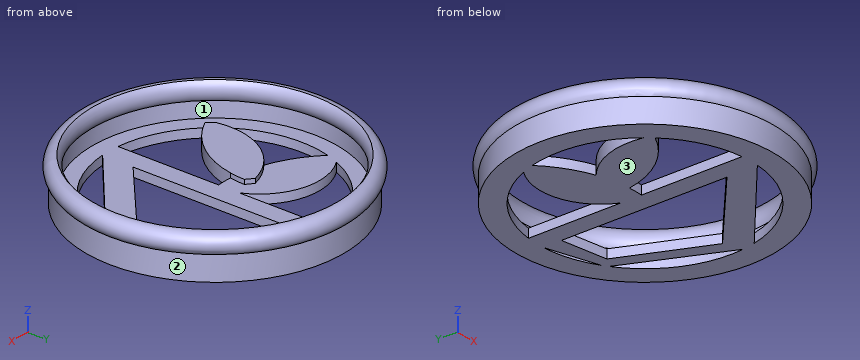
from build123d import *

# Parameters (mm, degrees)
F3_DEPTH = 2
F4_DEPTH = 1


# Not quite as in the source:
# - a feature names something its author has since deleted; it is built from what else it names


with BuildPart() as f1:
    # F0 (on Front) → F1 (revolve)
    with BuildSketch(Plane.XZ):
        Polygon((-29, 0), (-24, 0), (-24, 2), (-27.5, 2), (-27.5, 5.5), (-29, 5.5), align=None)
        with BuildLine():
            ThreePointArc((-27.5, 9.6169896424), (-29.7772258205, 8.1149302096), (-29, 5.5))
            Line((-29, 5.5), (-27.5, 5.5))
            ThreePointArc((-27.5, 5.5), (-26.6610115833, 7.5584948212), (-27.5, 9.6169896424))
        make_face()
    revolve(axis=Axis((0, 0, 2.7132770047), (0, 0, -1)))

    # F2 (on face) → F3 (join)
    with BuildSketch(Plane.XY.offset(2)):
        with BuildLine():
            Line((23.5357220544, -2.0133285341), (14.1158952872, 19.40982999))
            ThreePointArc((14.1158952872, 19.40982999), (13.5624984717, 19.8004705804), (12.9982976167, 20.1753378923))
            Line((12.9982976167, 20.1753378923), (1.5001369464, 23.9530705577))
            ThreePointArc((1.5001369464, 23.9530705577), (-0.61185618, 23.9921993993), (-2.7191094967, 23.8454700844))
            Line((-2.7191094967, 23.8454700844), (-2.7191094967, 3.205855377))
            Line((-2.7191094967, 3.205855377), (-2.7191094967, -1.398249995))
            Line((-2.7191094967, -1.398249995), (-2.7191094967, -23.8454700844))
            ThreePointArc((-2.7191094967, -23.8454700844), (-0.6587764532, -23.9909569127), (1.406435812, -23.9587549407))
            Line((1.406435812, -23.9587549407), (23.3430031088, -5.5771144744))
            ThreePointArc((23.3430031088, -5.5771144744), (23.6412294167, -4.1342800662), (23.8503615327, -2.6758652355))
            Line((23.8503615327, -2.6758652355), (23.5357220544, -2.0133285341))
        make_face()
        Polygon((1.5001369464, -17.0947052702), (1.5001369464, 19.8581963794), (11.7461745714, 17.9819713885), (19.9739150703, -1.2165056542), align=None, mode=Mode.SUBTRACT)
        with BuildLine():
            ThreePointArc((-2.7191094967, 3.205855377), (-11.036038033, 10.667911986), (-22.125575094, 9.2983292455))
            ThreePointArc((-22.125575094, 9.2983292455), (-22.6453594845, 7.9490687392), (-23.0829490937, 6.5709558771))
            ThreePointArc((-23.0829490937, 6.5709558771), (-14.7738683342, 6.6118059769), (-7.1936681304, 3.2084169794))
            ThreePointArc((-7.1936681304, 3.2084169794), (-6.4176007096, 2.6054477842), (-5.6727145132, 1.9643572708))
            ThreePointArc((-5.6727145132, 1.9643572708), (-4.0996738523, 0.3675861057), (-2.7191094967, -1.398249995))
            Line((-2.7191094967, -1.398249995), (-2.7191094967, 3.205855377))
        make_face()
        with BuildLine():
            ThreePointArc((-7.1936681304, 3.2084169794), (-14.7738683342, 6.6118059769), (-23.0829490937, 6.5709558771))
            ThreePointArc((-23.0829490937, 6.5709558771), (-18.5638120771, 2.8268811021), (-13.3236565945, 0.1846347444))
            ThreePointArc((-13.3236565945, 0.1846347444), (-10.4265323426, 2.0368417185), (-7.1936681304, 3.2084169794))
        make_face()
        with BuildLine():
            ThreePointArc((-13.3236565945, 0.1846347444), (-9.7250792571, -0.8614617254), (-6.0139401649, -1.3825407177))
            ThreePointArc((-6.0139401649, -1.3825407177), (-5.7755854856, 0.2840018043), (-5.6727145132, 1.9643572708))
            ThreePointArc((-5.6727145132, 1.9643572708), (-6.4176007096, 2.6054477842), (-7.1936681304, 3.2084169794))
            ThreePointArc((-7.1936681304, 3.2084169794), (-10.4265323426, 2.0368417185), (-13.3236565945, 0.1846347444))
        make_face()
        with BuildLine():
            ThreePointArc((-18.8341819929, -14.8752676836), (-18.1973718669, -15.6478642996), (-17.528892227, -16.3932283976))
            ThreePointArc((-17.528892227, -16.3932283976), (-9.9671253359, -10.2719865524), (-6.0139401649, -1.3825407177))
            ThreePointArc((-6.0139401649, -1.3825407177), (-9.7250792571, -0.8614617254), (-13.3236565945, 0.1846347444))
            ThreePointArc((-13.3236565945, 0.1846347444), (-18.1653516525, -6.5818760317), (-18.8341819929, -14.8752676836))
        make_face()
        with BuildLine():
            ThreePointArc((-6.0139401649, -1.3825407177), (-4.3667724447, -1.4423293633), (-2.7191094967, -1.398249995))
            ThreePointArc((-2.7191094967, -1.398249995), (-4.0996738523, 0.3675861057), (-5.6727145132, 1.9643572708))
            ThreePointArc((-5.6727145132, 1.9643572708), (-5.7755854856, 0.2840018043), (-6.0139401649, -1.3825407177))
        make_face()
    extrude(amount=-F3_DEPTH)

    # F2 (on face) → F4 (join)
    with BuildSketch(Plane.XY.offset(2)):
        with BuildLine():
            ThreePointArc((-18.8341819929, -14.8752676836), (-18.1973718669, -15.6478642996), (-17.528892227, -16.3932283976))
            ThreePointArc((-17.528892227, -16.3932283976), (-9.9671253359, -10.2719865524), (-6.0139401649, -1.3825407177))
            ThreePointArc((-6.0139401649, -1.3825407177), (-9.7250792571, -0.8614617254), (-13.3236565945, 0.1846347444))
            ThreePointArc((-13.3236565945, 0.1846347444), (-18.1653516525, -6.5818760317), (-18.8341819929, -14.8752676836))
        make_face()
        with BuildLine():
            ThreePointArc((-13.3236565945, 0.1846347444), (-9.7250792571, -0.8614617254), (-6.0139401649, -1.3825407177))
            ThreePointArc((-6.0139401649, -1.3825407177), (-5.7755854856, 0.2840018043), (-5.6727145132, 1.9643572708))
            ThreePointArc((-5.6727145132, 1.9643572708), (-6.4176007096, 2.6054477842), (-7.1936681304, 3.2084169794))
            ThreePointArc((-7.1936681304, 3.2084169794), (-10.4265323426, 2.0368417185), (-13.3236565945, 0.1846347444))
        make_face()
    extrude(amount=F4_DEPTH)


solid = f1.part
Read the model definition and answer for the solid it produces. Units are mm, in the model's axes. Face numbers are marked on the shaded views. Round coordinates to 2 decimals unless told otherwise and drop trailing zeros. Write each loop counter-clockwise with the first axis right and the second up, starting at its lowest first coordinate (ties: lowest second). Pieces come first, ordered by that corner, then holes.
Q1. Find section A-A on x = 0. Determine the outline of the cut face in (y, z), and give its area (3 significant figures).
Values:
outline: (-29, 0) - (29, 0) - (29, 5.5) arc R2.29 ccw to (27.5, 9.62) arc R2.94 ccw to (27.5, 5.5) - (27.5, 2) - (-27.5, 2) - (-27.5, 5.5) arc R2.94 ccw to (-27.5, 9.62) arc R2.29 ccw to (-29, 5.5) - close
area: 148 mm2
Q2. The mould has two halves that part along Y. Classify the marked faces 1, 2 and 3: released by +Y, released by -Y, zero draft, split by the parting line, or undercut.
Values:
face 1: undercut
face 2: split by the parting line
face 3: zero draft
Q3. Straight lines are drawn through the part: line 1 (Z direction, x = -4, y = 0); line 2 (X direction, y = -0.5, z = 3.75); line 3 (X direction, y = -19.5, z = 2.25). For each, find the intervals that lie inside material, in ascending order.
Values:
line 1: z = 0 to 2
line 2: x = -29 to -27.5, 27.5 to 29
line 3: x = -21.47 to -19.39, 19.39 to 21.47
Q4. Find section C-C on y = 16. State how many separate pieces and enclosed holes the cut face has, and give its area (3 significant figures).
Values:
separate pieces: 4
enclosed holes: 0
area: 78.4 mm2
Q5. Flat-ended cylindrical pins translate along their axes: P1, Ø2, axis at y = 23, z = 4.5, coming from the -X side; P2, Ø1.6, axis at y = -11, z = 1, coming from the -X side; P3, Ø1, axis at x = 0.5, z = 6.5, coming from the -Y side. Find the tip coordinate at first contact, or state that the pin passes through.
Values:
P1: stops at x = -18.89
P2: stops at x = -27.15
P3: stops at y = -29.89
Q6. Find section B-B on z = 4. Determine the outline of the cut face in (x, y), and give its area (3 significant figures).
Values:
outline: circle Ø58 at (0, 0); hole circle Ø55 at (0, 0)
area: 266 mm2
